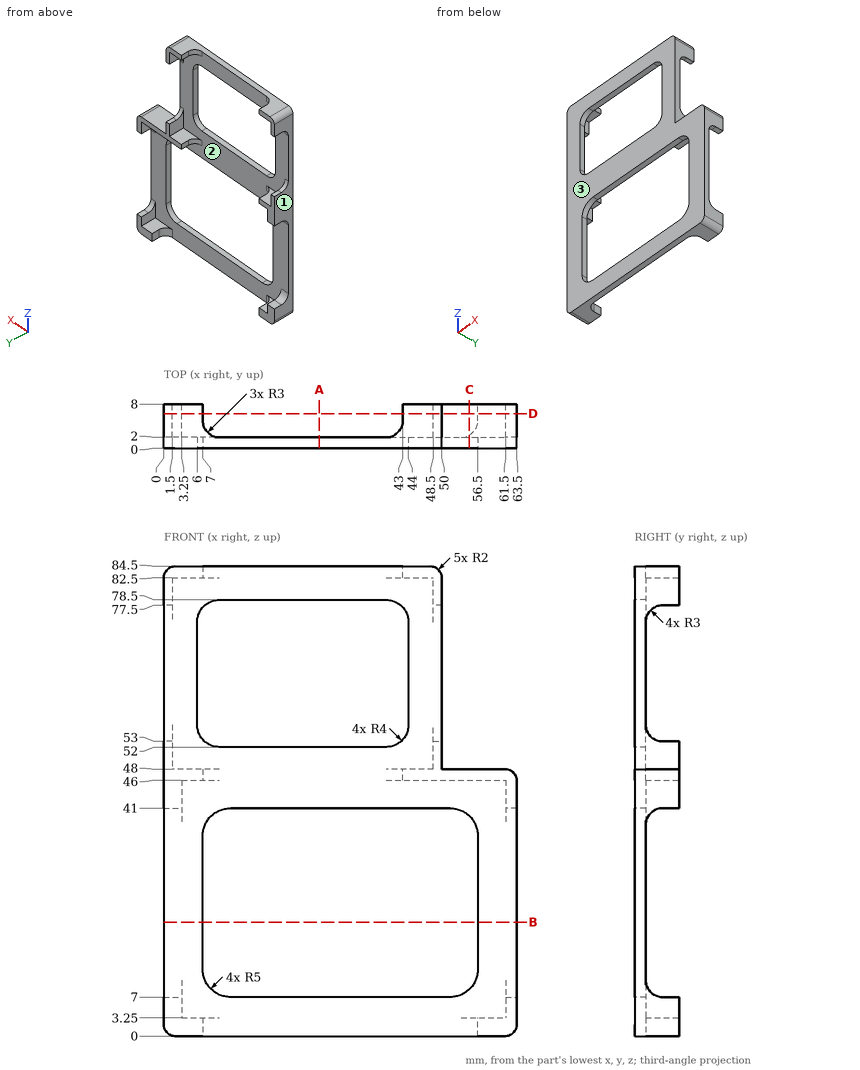
Here's the drawing with two shaded views (mm, measured from the low corner). I have some questions. Round coordinates to 2 decimals unless told otherwise and drop trailing zeros. Loops run counter-clockwise (first coordinate to the right, second up) from the corner with the lowest first, then second, coordinate; pieces in that order, holes last.
Item 1: Suppose I cut it at A-A, the plane x = 28. Write out the boundary of the cut face in (y, z), then the cut area to 3 significant figures.
Item 2: Suppose I cut it at C-C, the plane x = 55. Write out the boundary of the cut face in (y, z).
Item 3: Will these pins go through, and if not, where does the flat tip stop? pin 1 Ø2 at (y, z) = (1.5, 63.5) entering from +X; pin 2 Ø1.2 at (x, y) = (0.5, 6) entering from +Z; pin 3 Ø0.6 at (x, y) = (62.5, 6) entering from -Z.
Item 4: If we mould it in two halves opening along X, with no side actions, what happens to the marked faces 1, 2 and 3? For each: +X half, -X half, draft (parallel to the pull), parting line (faces both ways), or undercut.
Item 5: Suppose I cut it at B-B, the plane z = 20.5. Write out the boundary of the cut face in (x, y).
Item 6: Suppose I cut it at D-D, the plane y = 6.25. State how many separate pieces and enclosed holes the cut face has, then the cut area to 3 significant figures.
Item 7: Please list where these lines run through material, in increasing order: L1, parallel to Z at x = 17, y = 1; L2, parallel to Z at x = 58, y = 6.75; L3, parallel to Z at x = 5.5, y = 4.25.
Reported:
1. outline: (0, 0) - (2, 0) - (2, 7) - (0, 7) - close; (0, 41) - (2, 41) - (2, 52) - (0, 52) - close; (0, 78.5) - (2, 78.5) - (2, 84.5) - (0, 84.5) - close
1. area: 48.0 mm2
2. outline: (0, 0) - (2.4, 0) - (2.4, 3.25) - (2, 3.25) - (2, 8.43) - (0, 8.43) - close; (0, 39.57) - (2, 39.57) - (2, 46) - (8, 46) - (8, 48) - (0, 48) - close
3. pin 1: stops at x = 50
3. pin 2: stops at z = 84.29
3. pin 3: stops at z = 0.13
4. face 1: -X half
4. face 2: undercut
4. face 3: draft
5. outline: (0, 0) - (7, 0) - (7, 2) - (0, 2) - close; (56.5, 0) - (63.5, 0) - (63.5, 2) - (56.5, 2) - close
6. separate pieces: 6
6. enclosed holes: 0
6. area: 200 mm2
7. L1: z = 0 to 7, 41 to 52, 78.5 to 84.5
7. L2: z = 0 to 3.25, 46 to 48
7. L3: z = 0 to 3.25, 46 to 48, 82.5 to 84.5
